from build123d import *

# Parameters (mm, degrees)
F1_DEPTH = 25.4


with BuildPart() as f1:
    # F0 (on Right) → F1 (new body)
    with BuildSketch(Plane.YZ):
        with BuildLine():
            Line((5.3862427492, 76.7555311322), (0, 76.7555311322))
            Line((0, 76.7555311322), (0, 64.6187240932))
            ThreePointArc((0, 64.6187240932), (1.9314521574, 64.8609267634), (3.8662446042, 65.0748140172))
            ThreePointArc((3.8662446042, 65.0748140172), (4.5949489658, 70.9192449191), (5.3862427492, 76.7555311322))
        make_face()
        with BuildLine():
            Line((75.4848867655, 76.7555311322), (5.3862427492, 76.7555311322))
            ThreePointArc((5.3862427492, 76.7555311322), (4.5949489658, 70.9192449191), (3.8662446042, 65.0748140172))
            ThreePointArc((3.8662446042, 65.0748140172), (32.7930120665, 64.8934055874), (60.9952815162, 58.4573522376))
            ThreePointArc((60.9952815162, 58.4573522376), (68.191493841, 62.5298426374), (75.4848867655, 66.4256184947))
            Line((75.4848867655, 66.4256184947), (75.4848867655, 76.7555311322))
        make_face()
        with BuildLine():
            ThreePointArc((3.8662446042, 65.0748140172), (1.9314521574, 64.8609267634), (0, 64.6187240932))
            Line((0, 64.6187240932), (0, 13.0880264162))
            ThreePointArc((0, 13.0880264162), (0.0797042079, 13.1625355732), (0.1594323913, 13.2370190749))
            ThreePointArc((0.1594323913, 13.2370190749), (1.399759177, 39.199756565), (3.8662446042, 65.0748140172))
        make_face()
        with BuildLine():
            ThreePointArc((0.1594323913, 13.2370190749), (0.0797042079, 13.1625355732), (0, 13.0880264162))
            Line((0, 13.0880264162), (0, 0))
            ThreePointArc((0, 0), (0.0398595433, 6.6189895882), (0.1594323913, 13.2370190749))
        make_face()
        with BuildLine():
            Line((0, 0), (0, 13.0880264162))
            ThreePointArc((0, 13.0880264162), (-57.2227485948, -56.9347894415), (-93.8985440453, -139.5938707663))
            ThreePointArc((-93.8985440453, -139.5938707663), (-74.7023537588, -162.8329992856), (-50.7631260646, -181.1486809071))
            ThreePointArc((-50.7631260646, -181.1486809071), (134.418433918, -130.3074814993), (75.4848867655, 52.459787821))
            Line((75.4848867655, 52.459787821), (75.4848867655, 0))
            Line((75.4848867655, 0), (0, 0))
        make_face()
        with BuildLine():
            ThreePointArc((390.9781885196, 64.6620097575), (233.4491947056, 104.480650876), (75.4848867655, 66.4256184947))
            Line((75.4848867655, 66.4256184947), (75.4848867655, 52.459787821))
            ThreePointArc((75.4848867655, 52.459787821), (134.418433918, -130.3074814993), (-50.7631260646, -181.1486809071))
            ThreePointArc((-50.7631260646, -181.1486809071), (-57.3407742049, -218.7050554571), (-46.5994364643, -255.2888003165))
            ThreePointArc((-46.5994364643, -255.2888003165), (-15.8351680469, -347.0549469278), (75.9935366918, -316.4779153328))
            ThreePointArc((75.9935366918, -316.4779153328), (84.4804183959, -324.2078161859), (93.5921058689, -331.1903429243))
            ThreePointArc((93.5921058689, -331.1903429243), (99.5887961578, -335.1608026322), (105.7880268546, -338.8069490201))
            Line((105.7880268546, -338.8069490201), (390.9781885196, 64.6620097575))
        make_face()
        with BuildLine():
            Line((75.4848867655, 52.459787821), (75.4848867655, 66.4256184947))
            ThreePointArc((75.4848867655, 66.4256184947), (68.191493841, 62.5298426374), (60.9952815162, 58.4573522376))
            ThreePointArc((60.9952815162, 58.4573522376), (68.3286241876, 55.6724752477), (75.4848867655, 52.459787821))
        make_face()
        with BuildLine():
            Line((508.869806802, 231.447596607), (390.9781885196, 64.6620097575))
            ThreePointArc((390.9781885196, 64.6620097575), (466.8429069503, 9.5420995027), (524.7053222998, -64.2522153119))
            Line((524.7053222998, -64.2522153119), (530.5195744083, -59.0245212478))
            Line((530.5195744083, -59.0245212478), (553.822797689, -43.7876499609))
            Line((553.822797689, -43.7876499609), (579.178814564, -32.2865687022))
            Line((579.178814564, -32.2865687022), (605.9933014884, -24.7908530686))
            Line((605.9933014884, -24.7908530686), (625.8747293704, -22.4070069681))
            Line((625.8747293704, -22.4070069681), (508.869806802, 231.447596607))
        make_face()
        with BuildLine():
            ThreePointArc((524.7053222998, -64.2522153119), (466.8429069503, 9.5420995027), (390.9781885196, 64.6620097575))
            Line((390.9781885196, 64.6620097575), (105.7880268546, -338.8069490201))
            ThreePointArc((105.7880268546, -338.8069490201), (176.1168073384, -355.610653428), (245.0538575649, -333.7889909744))
            ThreePointArc((245.0538575649, -333.7889909744), (176.5880738948, -383.3985207357), (100.8892695091, -345.7374003159))
            Line((100.8892695091, -345.7374003159), (30.2667221668, -445.6497026059))
            Line((30.2667221668, -445.6497026059), (459.8510392405, -485.156246703))
            ThreePointArc((459.8510392405, -485.156246703), (510.8462412084, -426.6986552247), (547.2178651376, -358.1792740399))
            Line((547.2178651376, -358.1792740399), (531.7915045279, -348.2852703807))
            Line((531.7915045279, -348.2852703807), (510.9243750188, -329.8525449194))
            Line((510.9243750188, -329.8525449194), (493.1155417724, -308.4504908057))
            Line((493.1155417724, -308.4504908057), (478.7824287459, -284.5807540487))
            Line((478.7824287459, -284.5807540487), (468.2609919604, -258.8028210468))
            Line((468.2609919604, -258.8028210468), (461.7978449766, -231.7209047013))
            Line((461.7978449766, -231.7209047013), (459.5444784819, -203.9697821776))
            Line((459.5444784819, -203.9697821776), (461.5537094771, -176.1999162671))
            Line((461.5537094771, -176.1999162671), (467.7784432907, -149.0622090899))
            Line((467.7784432907, -149.0622090899), (478.0727774378, -123.1927455016))
            Line((478.0727774378, -123.1927455016), (492.1954214511, -99.1978838026))
            Line((492.1954214511, -99.1978838026), (509.8153525247, -77.640043214))
            Line((509.8153525247, -77.640043214), (524.7053222998, -64.2522153119))
        make_face()
        with BuildLine():
            Line((530.5195744083, -59.0245212478), (524.7053222998, -64.2522153119))
            ThreePointArc((524.7053222998, -64.2522153119), (569.58102559, -208.6407558217), (547.2178651376, -358.1792740399))
            Line((547.2178651376, -358.1792740399), (555.2278224701, -363.3166197278))
            Line((555.2278224701, -363.3166197278), (580.6840014165, -374.594270872))
            Line((580.6840014165, -374.594270872), (607.5633701083, -381.8538852288))
            Line((607.5633701083, -381.8538852288), (635.2358989253, -384.9253035909))
            Line((635.2358989253, -384.9253035909), (663.0529672461, -383.7365345149))
            Line((663.0529672461, -383.7365345149), (690.362566566, -378.3154417404))
            Line((690.362566566, -378.3154417404), (716.5245830234, -368.7890910874))
            Line((716.5245830234, -368.7890910874), (740.9258011265, -355.3807721411))
            Line((740.9258011265, -355.3807721411), (762.9942770044, -338.4047645331))
            Line((762.9942770044, -338.4047645331), (768.7441699807, -332.3774288358))
            Line((768.7441699807, -332.3774288358), (625.8747293704, -22.4070069681))
            Line((625.8747293704, -22.4070069681), (605.9933014884, -24.7908530686))
            Line((605.9933014884, -24.7908530686), (579.178814564, -32.2865687022))
            Line((579.178814564, -32.2865687022), (553.822797689, -43.7876499609))
            Line((553.822797689, -43.7876499609), (530.5195744083, -59.0245212478))
        make_face()
        with BuildLine():
            Line((100.8892695091, -345.7374003159), (105.7880268546, -338.8069490201))
            ThreePointArc((105.7880268546, -338.8069490201), (99.5887961578, -335.1608026322), (93.5921058689, -331.1903429243))
            ThreePointArc((93.5921058689, -331.1903429243), (96.8772664999, -338.6461726736), (100.8892695091, -345.7374003159))
        make_face()
        with BuildLine():
            ThreePointArc((245.0538575649, -333.7889909744), (176.1168073384, -355.610653428), (105.7880268546, -338.8069490201))
            Line((105.7880268546, -338.8069490201), (100.8892695091, -345.7374003159))
            ThreePointArc((100.8892695091, -345.7374003159), (176.5880738948, -383.3985207357), (245.0538575649, -333.7889909744))
        make_face()
        with BuildLine():
            Line((555.2278224701, -363.3166197278), (547.2178651376, -358.1792740399))
            ThreePointArc((547.2178651376, -358.1792740399), (510.8462412084, -426.6986552247), (459.8510392405, -485.156246703))
            Line((459.8510392405, -485.156246703), (855.9517264366, -521.5834826231))
            Line((855.9517264366, -521.5834826231), (768.7441699807, -332.3774288358))
            Line((768.7441699807, -332.3774288358), (762.9942770044, -338.4047645331))
            Line((762.9942770044, -338.4047645331), (740.9258011265, -355.3807721411))
            Line((740.9258011265, -355.3807721411), (716.5245830234, -368.7890910874))
            Line((716.5245830234, -368.7890910874), (690.362566566, -378.3154417404))
            Line((690.362566566, -378.3154417404), (663.0529672461, -383.7365345149))
            Line((663.0529672461, -383.7365345149), (635.2358989253, -384.9253035909))
            Line((635.2358989253, -384.9253035909), (607.5633701083, -381.8538852288))
            Line((607.5633701083, -381.8538852288), (580.6840014165, -374.594270872))
            Line((580.6840014165, -374.594270872), (555.2278224701, -363.3166197278))
        make_face()
        Polygon((633.6377496157, -21.4761962813), (625.8747293704, -22.4070069681), (768.7441699807, -332.3774288358), (782.212744287, -318.2589714936), (798.13073839, -295.4155933367), (810.3751550229, -270.4100594852), (818.658995438, -243.8284784588), (822.7880934368, -216.2938999874), (822.665666462, -188.4517112531), (818.2945840981, -160.9545095619), (809.7773008109, -134.4468060158), (797.3134545018, -109.5499187191), (781.1951871644, -86.8474096084), (761.8002973238, -66.8714062555), (739.5833847597, -50.0901292482), (715.0651950722, -36.8969174962), (688.8204138471, -27.6010087011), (661.4641965122, -22.4202910862), align=None)
    extrude(amount=F1_DEPTH)


solid = f1.part
The model under review builds one solid part; all positions refer to its coordinate system, in mm. A direction names the side the tool comes from. Give positions to 0.01 mm unless a question says otherwise; leave off trailing zeros. Order: outer loops, then holes, each group sorted by start corner. A loop starts at its lowest first (then second) coordinate and runs counter-clockwise, first axis right, second up. Notation, with made-up numbers: M -5.5,-37.5 L 46.5,-37.5 A15 cw 46.5,-19.5 Z; hole C 73.25,53 d5. An arc over 180 degrees is marked long. Answer in a Markdown table with one row per item. Add a question column.
1. Add section C-C on y = 328. State the section outline as (x, z) points.
2. Machinability: for faces 5 (the flat face through (12.522, 820.695, -230.254)), 6 (the flat face through (12.522, 702.127, -32.314)), 7 (the flat face through (13, 0, 45)), 8 (the flat face through (12.522, 472.854, -136.309)), which of the approach directions +Z, -Z, +X, -X, +Y, -Y give a long, thin tool a straight path to every point of the face, cutting with its end or side? Answer none if there is none.
3. For pin 1 Ø7.5 at (x, z) = (10, 15.5) entering from -Y; pin 2 Ø5 at (x, z) = (15, 69.5) entering from +Y; pin 3 Ø12 at (x, y) = (6, 577.5) entering from -Z, all flat-tipped, find the tip position at first contact; note any pin that passes through.
4. To check wall thickness, follow line 1 along Z through (x, y) = (15.25, 62.5); line 2 along Z through (x, y) = (1.5, 59.5); line 3 along Y through (x, z) = (20.5, -109). State the ranges of each line that lie inside material, in increasing order.
5. Add section B-B on y = 144. State the section outline as (x, z) points.
6. Mouldability with a two-part tool opening along Z and no side actions: class faces 1 (the flat face through (13, 38, 0)), 2 (the flat face through (12.522, 771.634, -76.999)), 3 (the flat face through (12.522, 437.329, -483.085)), 4 (the flat face through (12.522, 804.167, -283.088)) as released by +Z, released by -Z, zero draft, split by the parting line, or undercut.
7. Add section A-A on x = 16. Count the separate pieces of the cut face and the enclosed holes in it, plus the area to 3 significant figures.
The answers:
| question | item | result |
|---|---|---|
| 1 | outline | M 0,-473.03 L 25.4,-473.03 L 25.4,90.48 L 0,90.48 Z |
| 2 | face 5 | +X, -X, +Y |
| 2 | face 6 | +Z, +X, -X, +Y |
| 2 | face 7 | +Z, +X, -X, -Y |
| 2 | face 8 | +X, -X |
| 3 | pin 1 | y = -1.42 |
| 3 | pin 2 | y = 584.67 |
| 3 | pin 3 | z = -496.53 |
| 4 | line 1 | -448.61 to -400.05, -334.89 to 0, 57.93 to 76.76 |
| 4 | line 2 | -448.34 to -404.29, -337.64 to 0, 58.97 to 76.76 |
| 4 | line 3 | -83.37 to 486.43, 546.47 to 796.92 |
| 5 | outline | M 0,-456.11 L 25.4,-456.11 L 25.4,92.99 L 0,92.99 Z |
| 6 | face 1 | undercut |
| 6 | face 2 | released by +Z |
| 6 | face 3 | released by -Z |
| 6 | face 4 | undercut |
| 7 | separate pieces | 1 |
| 7 | enclosed holes | 2 |
| 7 | area | 431,000 mm2 |
